Read the model definition and answer for the solid it produces. Units are mm, in the model's axes. Face numbers are marked on the shaded views. A direction names the side the tool comes from. Give positions to 0.01 mm unless a question says otherwise; leave off trailing zeros. Write each loop counter-clockwise with the first axis right and the second up, starting at its lowest first coordinate (ties: lowest second). Pieces come first, ordered by that corner, then holes. Notation, with made-up numbers: (56, 55) -> (79, 55) arc R23 cw to (79, 70) -> close; hole circle Ø4 at (-30, 31). An arc over 180 degrees is marked (long way). Write item = value, one per line.
from build123d import *

# Parameters (mm, degrees)
F1_DEPTH = 3.175
F2_R     = 6.35
F2_R_2   = 3.937
F3_DEPTH = 5.08
F4_R     = 12.7
F4_R_2   = 1.143
F4_R_3   = 3.937
F5_DEPTH = 5.08
F6_R     = 0.41275
F7_DEPTH = 5.0814106062


with BuildPart() as f1:
    # F0 (on Right) → F1 (new body)
    with BuildSketch(Plane.YZ):
        with BuildLine():
            Line((-18.415, 5.1269156738), (-13.335, 5.1269156738))
            Line((-13.335, 5.1269156738), (-13.335, 29.1074568056))
            ThreePointArc((-13.335, 29.1074568056), (-13.1820577877, 30.4927274565), (-12.7305984957, 31.8112685458))
            Line((-12.7305984957, 31.8112685458), (-6.086145584, 45.930727414))
            ThreePointArc((-6.086145584, 45.930727414), (-3.7429944023, 48.5884315299), (-0.3405470883, 49.5769156738))
            Line((-0.3405470883, 49.5769156738), (0, 49.5769156738))
            Line((0, 49.5769156738), (0.3405470883, 49.5769156738))
            ThreePointArc((0.3405470883, 49.5769156738), (3.7429944023, 48.5884315299), (6.086145584, 45.930727414))
            Line((6.086145584, 45.930727414), (12.7305984957, 31.8112685458))
            ThreePointArc((12.7305984957, 31.8112685458), (13.1820577877, 30.4927274565), (13.335, 29.1074568056))
            Line((13.335, 29.1074568056), (13.335, 5.1269156738))
            Line((13.335, 5.1269156738), (18.415, 5.1269156738))
            Line((18.415, 5.1269156738), (18.415, 30.2430239001))
            ThreePointArc((18.415, 30.2430239001), (18.2620577877, 31.628294551), (17.8105984957, 32.9468356404))
            Line((17.8105984957, 32.9468356404), (9.3099413945, 51.010727414))
            ThreePointArc((9.3099413945, 51.010727414), (6.9667902129, 53.6684315299), (3.5643428989, 54.6569156738))
            Line((3.5643428989, 54.6569156738), (0, 54.6569156738))
            Line((0, 54.6569156738), (-3.5643428989, 54.6569156738))
            ThreePointArc((-3.5643428989, 54.6569156738), (-6.9667902129, 53.6684315299), (-9.3099413945, 51.010727414))
            Line((-9.3099413945, 51.010727414), (-17.8105984957, 32.9468356404))
            ThreePointArc((-17.8105984957, 32.9468356404), (-18.2620577877, 31.628294551), (-18.415, 30.2430239001))
            Line((-18.415, 30.2430239001), (-18.415, 5.1269156738))
        make_face()
    extrude(amount=F1_DEPTH)

    # F2 (on face) → F3 (join, through all)
    with BuildSketch(Plane.XZ.offset(18.415)):
        with Locations((1.5875, 1.1899156738)):
            Circle(F2_R)
        with Locations((1.5875, 1.1899156738)):
            Circle(F2_R_2, mode=Mode.SUBTRACT)
    extrude(amount=-F3_DEPTH)

    # F4 (on face) → F5 (join, through all)
    with BuildSketch(Plane(origin=(0, 18.415, 0), x_dir=(-1, 0, 0), z_dir=(0, 1, 0))):
        with Locations((-1.5875, 1.1899156739)):
            Circle(F4_R)
        with Locations((-11.1125, 1.1899156739)):
            Circle(F4_R_2, mode=Mode.SUBTRACT)
        with Locations((-1.5875, 1.1899156739)):
            Circle(F4_R_3, mode=Mode.SUBTRACT)
        with Locations((7.9375, 1.1899156739)):
            Circle(F4_R_2, mode=Mode.SUBTRACT)
    extrude(amount=-F5_DEPTH)

    # F6 (on face) → F7 (cut, through all)
    with BuildSketch(Plane.XY.offset(54.6569156738)):
        with Locations((1.5875, 0)):
            Circle(F6_R)
    extrude(amount=-F7_DEPTH, mode=Mode.SUBTRACT)


solid = f1.part
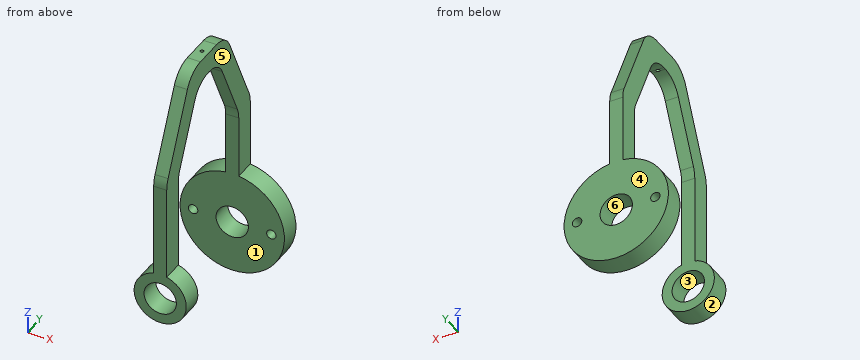
(1) For a pull along X with two mould halves and no side action, classify the marked faces 4, 5 and 6 as released by +X, released by -X, zero draft, split by the parting line, or undercut.
Checks:
face_4 = zero draft
face_5 = released by +X
face_6 = undercut
(2) The part is cut by section A-A on z = 28. Determine the outline of the cut face in (x, y) (3 decimals), plus the area to 3 significant figures.
Checks:
outline = (0, -18.415) -> (3.175, -18.415) -> (3.175, -13.335) -> (0, -13.335) -> close; (0, 13.335) -> (3.175, 13.335) -> (3.175, 18.415) -> (0, 18.415) -> close
area = 32.3 mm²
(3) A tool of negligible diameter and unlimited length cuts with its end or side. For the marked faces 1, 2 and 3, from which of +Z, -Z, +X, -X, +Y, -Y can it reach the whole face along a straight path? Write none if from no direction.
Checks:
face_1 = -Z, +X, -X
face_2 = -Y
face_3 = +Y, -Y
(4) Given P1, Ø5, axis at x = 11, z = 11, coming from the -Y side (3 decimals); P2, Ø18.5, axis at y = -3, z = 39, coming from the +X side (3 decimals); P3, Ø0.7, axis at x = 2.5, y = 0, coming from the -Z side, each flat-ended and moving along its own axis, determine where each tip first touches the part or whether it passes through.
Checks:
P1 = 13.335
P2 = 3.175
P3 = 49.58
(5) The part is cut by section C-C on y = -7. Determine the outline of the cut face in (x, z) (3 decimals).
Checks:
outline = (0, 43.989) -> (3.175, 43.989) -> (3.175, 53.647) -> (0, 53.647) -> close
(6) The part is cut by section B-B on x = -3.75. Determine the outline of the cut face in (y, z) (3 decimals), plus the area to 3 significant figures.
Checks:
outline = (-18.415, -2.25) -> (-13.335, -2.25) -> (-13.335, 4.63) -> (-18.415, 4.63) -> close; (13.335, -10.334) -> (18.415, -10.334) -> (18.415, 12.714) -> (13.335, 12.714) -> close
area = 152 mm²
(7) Consider L1, parallel to X at y = 17, z = 0.5; L2, parallel to X at y = 0, z = 51.15 (3 decimals); L3, parallel to Y at x = 7, z = -0.5 (3 decimals). Determine where each line is inside the solid, lowest interval first.
Checks:
L1 = -11.09 to -8.85, -7.03 to -2.29, 5.46 to 10.2, 12.02 to 14.27
L2 = 0 to 1.175, 2 to 3.175
L3 = -18.415 to -13.335, 13.335 to 18.415
(8) The part is cut by section D-D on y = 7.5. Determine the outline of the cut face in (x, z) (3 decimals), plus the area to 3 significant figures.
Checks:
outline = (0, 42.926) -> (3.175, 42.926) -> (3.175, 53.29) -> (0, 53.29) -> close
area = 32.9 mm²
